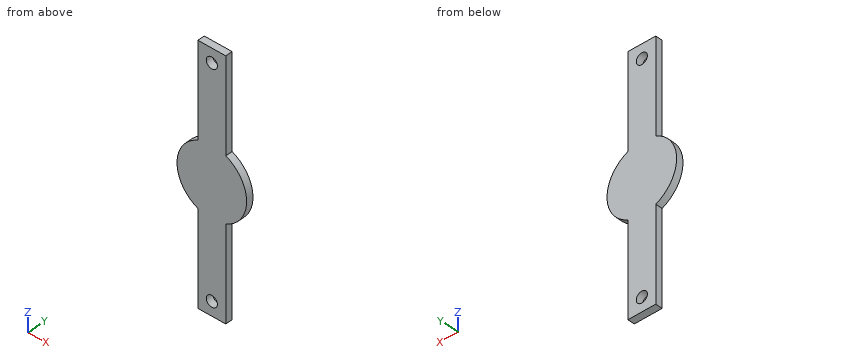
Autodesk Inventor part; units mm, degrees
ref_plane "YZ Plane" through (0, 0, 0) normal (1, 0, 0) x (0, 1, 0)
ref_plane "XZ Plane" through (0, 0, 0) normal (0, 1, 0) x (-1, 0, 0)
ref_plane "XY Plane" through (0, 0, 0) normal (0, 0, 1) x (1, 0, 0)
sketch "Boceto1" plane through (0, 0, 0) normal (0, 1, 0) x (-1, 0, 0)
  line L0 (10, 90) -> (-10, 90)
  line L1 (-10, 90) -> (-10, -90)
  line L2 (-10, -90) -> (10, -90)
  line L3 (10, -90) -> (10, 90)
  line L4 (14, 0) -> (-14, 0)
  line L5 (0, -126) -> (0, 126)
  point P0 (0, 0)
  point P1 (10, 0)
  point P2 (0, 90)
  dimension "d0" = 20
  dimension "d1" = 180
extrude "Extrusión1" add sketch "Boceto1" along normal blind 5
sketch "Boceto2" plane through (0, 5, 0) normal (0, 1, 0) x (1, 0, 0)
  line L0 (10, 90) -> (-10, 90)
  line L1 (-10, 90) -> (-10, -90)
  line L2 (-10, -90) -> (10, -90)
  line L3 (10, -90) -> (10, 90)
  circle A0 centre (0, -80) radius 4
  circle A1 centre (0, 80) radius 4
  line L4 (0, 126) -> (0, -126)
  point P0 (0, 0)
  dimension "d4" = 8
  dimension "d5" = 8
  dimension "d6" = 10
  dimension "d7" = 10
extrude "Extrusión2" cut sketch "Boceto2" against normal blind 5 contours L4 A1 | A1 L4 | L4 A0 | A0 L4
sketch "Boceto3" plane through (0, 5, 0) normal (0, 1, 0) x (1, 0, 0)
  circle A0 centre (0, 0) radius 25
  dimension "d10" = 50
extrude "Extrusión3" add sketch "Boceto3" against normal blind 5
equation "\"d5\" = d4"
properties part number "PlacaRetencion"
Check sheet for the modelled part. Datum: model origin and axes. Units: mm. Round coordinates to 2 decimals unless told otherwise and drop trailing zeros. Loops run counter-clockwise (first coordinate to the right, second up) from the corner with the lowest first, then second, coordinate; pieces in that order, holes last.
1. Scan lines: probe 1 along Z at (x, y) = (0, 1.9); probe 2 along X at (y, z) = (3.55, -80); probe 3 along X at (y, z) = (2.3, 55). Record each from-to range of solid material in increasing order.
2. Sectioned sample at A-A on z = 80. Record the boundary of the cut face in (x, y).
3. Sectioned sample at C-C on y = 0.9. Record the boundary of the cut face in (x, z), and give its area (3 significant figures).
4. Sectioned sample at B-B on x = 0. Record the boundary of the cut face in (y, z), and give its area (3 significant figures).
5. Gauge pin test, flat end, axial feed: pin 1 Ø3 at (y, z) = (2, -47.5) entering from +X. Record the tip position at first contact, or that the pin passes through.
6. Sectioned sample at D-D on x = -18.5. Record the boundary of the cut face in (y, z), and give its area (3 significant figures).
Recorded:
1. probe 1: z = -90 to -84, -76 to 76, 84 to 90
1. probe 2: x = -10 to -4, 4 to 10
1. probe 3: x = -10 to 10
2. outline: (-10, 0) - (-4, 0) - (-4, 5) - (-10, 5) - close; (4, 0) - (10, 0) - (10, 5) - (4, 5) - close
3. outline: (-10, -90) - (10, -90) - (10, -22.91) arc R25 ccw to (10, 22.91) - (10, 90) - (-10, 90) - (-10, 22.91) arc R25 ccw to (-10, -22.91) - close; hole circle Ø8 at (0, -80); hole circle Ø8 at (0, 80)
3. area: 4,490 mm2
4. outline: (0, -90) - (5, -90) - (5, -84) - (0, -84) - close; (0, -76) - (5, -76) - (5, 76) - (0, 76) - close; (0, 84) - (5, 84) - (5, 90) - (0, 90) - close
4. area: 820 mm2
5. pin 1: stops at x = 10
6. outline: (0, -16.82) - (5, -16.82) - (5, 16.82) - (0, 16.82) - close
6. area: 168 mm2
